```python
from build123d import *

# Parameters (mm, degrees)
CROQUIS1_R              = 2.1
SALIENTE_EXTRUIR2_DEPTH = 300


with BuildPart() as part:
    # Croquis1 → Saliente-Extruir2 (new body)
    with BuildSketch(Plane(origin=(0, 0, 0), x_dir=(1, 0, 0), z_dir=(0, 1, 0))):
        with BuildLine():
            Line((3.9, -2.84), (3.9, 2.84))
            Line((3.9, 2.84), (6.36, 5.3))
            Line((6.36, 5.3), (8.2, 5.3))
            Line((8.2, 5.3), (8.2, 3.34))
            ThreePointArc((8.2, 3.34), (8.346446609, 2.986446609), (8.7, 2.84))
            Line((8.7, 2.84), (10, 4.14))
            Line((10, 4.14), (10, 8))
            ThreePointArc((10, 8), (9.414213562, 9.414213562), (8, 10))
            Line((8, 10), (4.14, 10))
            Line((4.14, 10), (2.84, 8.7))
            ThreePointArc((2.84, 8.7), (2.986446609, 8.346446609), (3.34, 8.2))
            Line((3.34, 8.2), (5.3, 8.2))
            Line((5.3, 8.2), (5.3, 6.36))
            Line((5.3, 6.36), (2.84, 3.9))
            Line((2.84, 3.9), (-2.84, 3.9))
            Line((-2.84, 3.9), (-5.3, 6.36))
            Line((-5.3, 6.36), (-5.3, 8.2))
            Line((-5.3, 8.2), (-3.34, 8.2))
            ThreePointArc((-3.34, 8.2), (-2.986446609, 8.346446609), (-2.84, 8.7))
            Line((-2.84, 8.7), (-4.14, 10))
            Line((-4.14, 10), (-8, 10))
            ThreePointArc((-8, 10), (-9.414213562, 9.414213562), (-10, 8))
            Line((-10, 8), (-10, 4.14))
            Line((-10, 4.14), (-8.7, 2.84))
            ThreePointArc((-8.7, 2.84), (-8.346446609, 2.986446609), (-8.2, 3.34))
            Line((-8.2, 3.34), (-8.2, 5.3))
            Line((-8.2, 5.3), (-6.36, 5.3))
            Line((-6.36, 5.3), (-3.9, 2.84))
            Line((-3.9, 2.84), (-3.9, -2.84))
            Line((-3.9, -2.84), (-6.36, -5.3))
            Line((-6.36, -5.3), (-8.2, -5.3))
            Line((-8.2, -5.3), (-8.2, -3.34))
            ThreePointArc((-8.2, -3.34), (-8.346446609, -2.986446609), (-8.7, -2.84))
            Line((-8.7, -2.84), (-10, -4.14))
            Line((-10, -4.14), (-10, -8))
            ThreePointArc((-10, -8), (-9.414213562, -9.414213562), (-8, -10))
            Line((-8, -10), (-4.14, -10))
            Line((-4.14, -10), (-2.84, -8.7))
            ThreePointArc((-2.84, -8.7), (-2.986446609, -8.346446609), (-3.34, -8.2))
            Line((-3.34, -8.2), (-5.3, -8.2))
            Line((-5.3, -8.2), (-5.3, -6.36))
            Line((-5.3, -6.36), (-2.84, -3.9))
            Line((-2.84, -3.9), (2.84, -3.9))
            Line((2.84, -3.9), (5.3, -6.36))
            Line((5.3, -6.36), (5.3, -8.2))
            Line((5.3, -8.2), (3.34, -8.2))
            ThreePointArc((3.34, -8.2), (2.986446609, -8.346446609), (2.84, -8.7))
            Line((2.84, -8.7), (4.14, -10))
            Line((4.14, -10), (8, -10))
            ThreePointArc((8, -10), (9.414213562, -9.414213562), (10, -8))
            Line((10, -8), (10, -4.14))
            Line((10, -4.14), (8.7, -2.84))
            ThreePointArc((8.7, -2.84), (8.346446609, -2.986446609), (8.2, -3.34))
            Line((8.2, -3.34), (8.2, -5.3))
            Line((8.2, -5.3), (6.36, -5.3))
            Line((6.36, -5.3), (3.9, -2.84))
        make_face()
        Circle(CROQUIS1_R, mode=Mode.SUBTRACT)
    extrude(amount=SALIENTE_EXTRUIR2_DEPTH)


solid = part.part
```
For this review, take the finished solid that the model builds, in its own axes (mm). A direction names the side the tool comes from. Give positions to 0.01 mm unless a question says otherwise; leave off trailing zeros.
Item 1: Machinability: for faces 5 (the face through (-0.1, 0, -2.4)), 6 (the face through (3.9, 148, 0)), which of the approach directions +Z, -Z, +X, -X, +Y, -Y give a long, thin tool a straight path to every point of the face, cutting with its end or side? Answer none if there is none.
Item 2: Wall thickness on probe 1 along X at (y, z) = (58.5, -5.25); probe 2 along Z at (x, y) = (0, 229.5); probe 3 along Z at (x, y) = (3.75, 127): over which ranges is each line inside the solid? List them lowest first.
Item 3: The part is to be moulded in two halves that separate along X. For faces 1 (the face through (-3.9, 148, 0)), 2 (the face through (-0.1, 300, -2.4)), 3 (the face through (0, 148, 3.9)), 4 (the face through (0, 148, -3.9)), say which applies: +X half, -X half, draft (parallel to the pull), parting line (faces both ways), or undercut.
Item 4: Insertion check: P1, Ø6, axis at x = 0.5, y = 151, coming from the -Z side; P2, Ø4.5, axis at y = 109.5, z = 0, coming from the +X side; P3, Ø3, axis at y = 95.5, z = 0.5, coming from the -X side. Each pin has a flat end and moves straight along its axis. Give the tip position at first contact, or say it passes through.
Established:
1. face 5: +Z, -Z, +X, -X, -Y
1. face 6: +X, +Y, -Y
2. probe 1: x = -10 to -8.2, -6.31 to -4.19, 4.19 to 6.31, 8.2 to 10
2. probe 2: z = -3.9 to -2.1, 2.1 to 3.9
2. probe 3: z = -9.61 to -8.2, -4.81 to 4.81, 8.2 to 9.61
3. face 1: -X half
3. face 2: draft
3. face 3: undercut
3. face 4: undercut
4. P1: stops at z = -9.36
4. P2: stops at x = 3.9
4. P3: stops at x = -3.9
